Check sheet for the drawn part. Datum: minimum x, y, z corner. Units: mm. Round coordinates to 2 decimals unless told otherwise and drop trailing zeros. Order: outer loops, then holes, each group sorted by start corner. A loop starts at its lowest first (then second) coordinate and runs counter-clockwise, first axis right, second up. Notation, with made-up numbers: (28, -12) -> (45, -12) arc R5 ccw to (45, -5) -> close; hole circle Ø9 at (30, -19.5). An arc over 180 degrees is marked (long way). Write item = value, one per line. Start each with the question number.
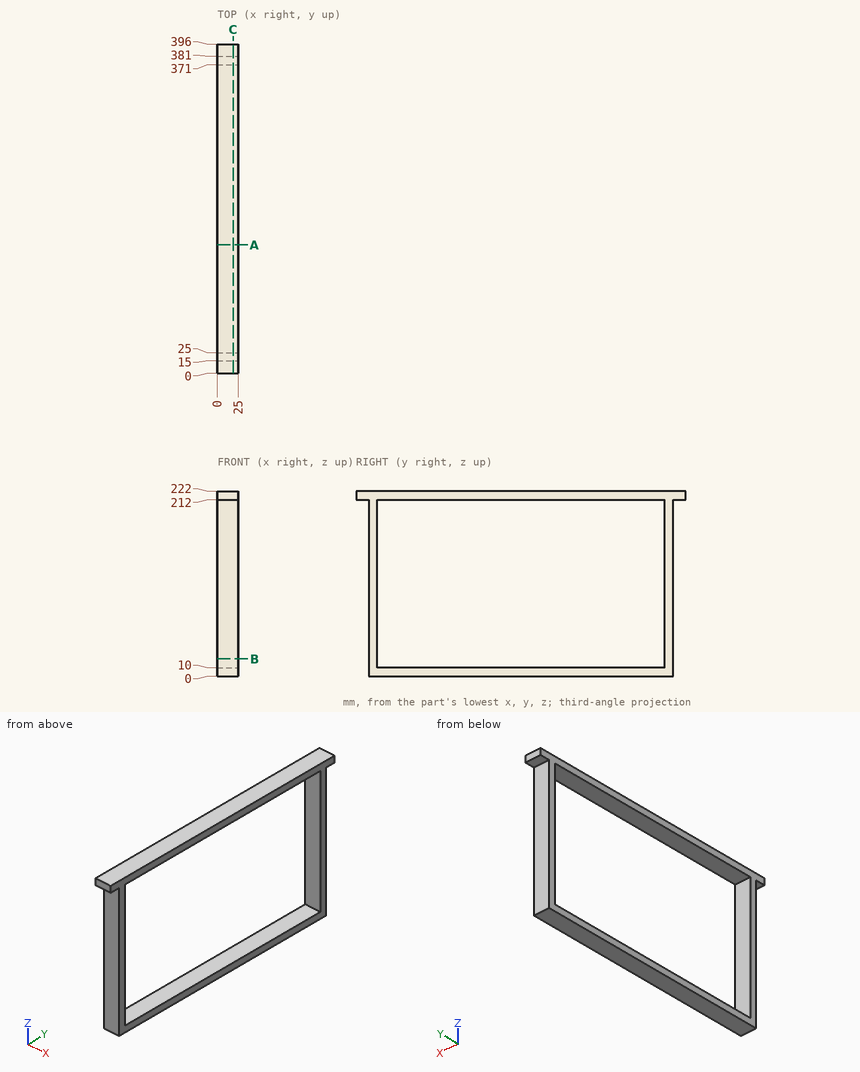
(1) Scan lines: line 1 along Y through (x, z) = (22.25, 132); line 2 along Z through (x, y) = (20.75, 222). Record each from-to range of solid material in increasing order. Write a range as from..to.
(2) Cross-section at B-B (z = 20.5). Enter the section's corners in (x, y).
(3) Cross-section at A-A (y = 154.5). Enter the section's corners in (x, z).
(4) Depth check by flat-ended pin: pin 1 (5 mm diameter, centred on x = 8, z = 134, fed in from +Y); pin 2 (7.5 mm diameter, centred on x = 14, z = 89.5, fed in from -Y); pin 3 (12.5 mm diameter, centred on x = 9, y = 157, fed in from -Z); pin 4 (12 mm diameter, centred on x = 10.5, y = 391, fed in from -Z). Enter the tip coordinate at first touch or a pass-through.
(5) Cross-section at C-C (x = 19). Enter the section's corners in (y, z).
Outcome:
q1.line_1 = 15..25, 371..381
q1.line_2 = 0..10, 212..222
q2.outline = (0, 15) -> (25, 15) -> (25, 25) -> (0, 25) -> close; (0, 371) -> (25, 371) -> (25, 381) -> (0, 381) -> close
q3.outline = (0, 0) -> (25, 0) -> (25, 10) -> (0, 10) -> close; (0, 212) -> (25, 212) -> (25, 222) -> (0, 222) -> close
q4.pin_1 = 381
q4.pin_2 = 15
q4.pin_3 = 0
q4.pin_4 = 212
q5.outline = (0, 212) -> (15, 212) -> (15, 0) -> (381, 0) -> (381, 212) -> (396, 212) -> (396, 222) -> (0, 222) -> close; hole (25, 10) -> (371, 10) -> (371, 212) -> (25, 212) -> close
